from build123d import *

# Parameters (mm, degrees)
EXTRUDE_1_DEPTH = 20


with BuildPart() as part:
    # 草图1 → 凸台-拉伸1 (new body)
    with BuildSketch(Plane(origin=(0, 0, 0), x_dir=(1, 0, 0), z_dir=(0, 1, 0))):
        with BuildLine():
            Line((-800, 400), (800, 400))
            ThreePointArc((800, 400), (835.355339059, 385.355339059), (850, 350))
            Line((850, 350), (850, -350))
            ThreePointArc((850, -350), (835.355339059, -385.355339059), (800, -400))
            Line((800, -400), (-800, -400))
            ThreePointArc((-800, -400), (-835.355339059, -385.355339059), (-850, -350))
            Line((-850, -350), (-850, 350))
            ThreePointArc((-850, 350), (-835.355339059, 385.355339059), (-800, 400))
        make_face()
    extrude(amount=EXTRUDE_1_DEPTH)

    # 扫描1: sweep along a path in 草图4
    with BuildLine(Plane(origin=(0, 20, 0), x_dir=(1, 0, 0), z_dir=(0, 1, 0))) as sweep_1_path:
        Line((800, 400), (-800, 400))
        ThreePointArc((-800, 400), (-835.355339059, 385.355339059), (-850, 350))
        Line((-850, 350), (-850, -350))
        ThreePointArc((-850, -350), (-835.355339059, -385.355339059), (-800, -400))
        Line((-800, -400), (800, -400))
        ThreePointArc((800, -400), (835.355339059, -385.355339059), (850, -350))
        Line((850, -350), (850, 350))
        ThreePointArc((850, 350), (835.355339059, 385.355339059), (800, 400))
    # 草图3 → 扫描1 (sweep)
    with BuildSketch(Plane(origin=(0, 0, 350), x_dir=(0, -1, 0), z_dir=(0, 0, 1))):
        with BuildLine():
            Line((0, 850), (-60, 850))
            Line((-60, 850), (-70, 877.474774195))
            Line((-70, 877.474774195), (-70, 915))
            Line((-70, 915), (-50, 915))
            ThreePointArc((-50, 915), (-35.355339059, 879.644660941), (0, 865))
            Line((0, 865), (0, 850))
        make_face()
    sweep(path=sweep_1_path.line)


solid = part.part
Can you work these out from the model? Positions are in its coordinate system, mm. A direction names the side the tool comes from. Coordinates: 2 decimals unless noted, no trailing zeros. Answer as a JSON object with one key per item and string values. Group by question number.
Q1. On a 3-axis mill with a long thin cutter (end or side, diameter ignored), from which of +Z, -Z, +X, -X, +Y, -Y can I reach the whole of each face in a straight line? I mean faces 4 (the face through (-880.418, 60.14, -432.206)), 5 (the face through (-835.742, 39.72, 384.964)). Say none if no direction works.
Q2. Will these pins go through, and if not, where does the flat tip stop? P1, Ø3, axis at x = -402.5, y = 41, coming from the +Z side; P2, Ø10, axis at x = 463.5, z = -13.5, coming from the +Y side; P3, Ø3, axis at y = 38, z = 274, coming from the -X side.
Q3. I need wall thicknesses on line 1 (Z direction, x = 206, y = 51); line 2 (Y direction, x = 168.5, z = -235); line 3 (X direction, y = 46, z = -236.5). Which ranges of each line are inside material? Lowest first, please. Write a range as from..to.
Q4. We'd pull the mould along Z, two halves only. Please class faces 1 (the face through (879.258, 34.964, -4.9)), 2 (the face through (880.418, 60.14, 432.206)), 3 (the face through (850, 40, -5)): +Z half, -Z half, draft (parallel to the pull), parting line (faces both ways), or undercut.
Determined:
{
 "1": {"face 4": "-Z, -X, +Y, -Y", "face 5": "+Y"},
 "2": {"P1": "stops at z = 438.66", "P2": "stops at y = 20", "P3": "stops at x = -884.34"},
 "3": {"line 1": "z = -465..-400, 400..465", "line 2": "y = 0..20", "line 3": "x = -895.4..-850, 850..895.4"},
 "4": {"face 1": "draft", "face 2": "+Z half", "face 3": "undercut"}
}
